Geometry check sheet. Reference: the model listing, model coordinates, mm. Face numbers are marked on the shaded views. A direction names the side the tool comes from. Give positions to 0.01 mm unless a question says otherwise; leave off trailing zeros. Write each loop counter-clockwise with the first axis right and the second up, starting at its lowest first coordinate (ties: lowest second). Pieces come first, ordered by that corner, then holes. Notation, with made-up numbers: M 85.5,-35 L 136.5,-35 A26 cw 136.5,-17 Z; hole C 51,10 d2. An arc over 180 degrees is marked long. One line per item, written item: value. Start each with the question number.
1. Scan lines: line 1 (X direction, y = 54, z = -15); line 2 (Y direction, x = 11, z = -24.5); line 3 (Z direction, x = 13.25, y = 60). Record each from-to range of solid material in increasing order.
2. Gauge pin test, flat ends, axial feed: pin 1 (1 mm diameter, centred on y = 41.5, z = -19, fed in from +X); pin 2 (10 mm diameter, centred on x = 13.5, y = 56.5, fed in from +Z); pin 3 (1.5 mm diameter, centred on x = 20, y = 50, fed in from +Z). Record the tip position at first contact, or that the pin passes through.
3. Tool access check on the marked faces 4 and 5. Record the directions out of +Z, -Z, +X, -X, +Y, -Y that give a thin tool (end or side, any length) a straight path to the whole face; none if there is none.
4. Cross-section at A-A on x = 15. Record the cut outline in (y, z), then the cut area to 3 significant figures.
5. Cross-section at C-C on x = 26. Record the cut outline in (y, z), then the cut area to 3 significant figures.
6. Cross-section at B-B on z = -26. Record the cut outline in (x, y), then the cut area to 3 significant figures.
7. Cross-section at D-D on z = -10.25. Record the cut outline in (x, y).
8. Release check for a two-part mould opening along X. For the marked faces 1, 2 and 3 record: pulls with the +X half, pulls with the -X half, needs draft (parallel to the pull), parting line crosses it, or undercut.
from build123d import *

# Parameters (mm, degrees)
IZIM1_W                     = 30
IZIM1_H                     = 30
Y_KSEKLIK_EKSTR_ZYON1_DEPTH = 40
IZIM2_R                     = 1.5
KES_EKSTR_ZYON1_DEPTH       = 40
IZIM3_R                     = 10
IZIM3_R_2                   = 5.25
Y_KSEKLIK_EKSTR_ZYON2_DEPTH = 40
IZIM4_W                     = 30
IZIM4_H                     = 30
KES_EKSTR_ZYON2_DEPTH       = 32
KES_EKSTR_ZYON3_START       = -10
IZIM5_R                     = 10
KES_EKSTR_ZYON3_DEPTH       = 10
KES_EKSTR_ZYON4_START       = -30
IZIM6_R                     = 5.25
KES_EKSTR_ZYON4_DEPTH       = 30


with BuildPart() as part:
    # Çizim1 → Yükseklik-Ekstrüzyon1 (new body)
    with BuildSketch(Plane(origin=(0, 0, 0), x_dir=(1, 0, 0), z_dir=(0, 1, 0))):
        with Locations((15, 15)):
            Rectangle(IZIM1_W, IZIM1_H)
    extrude(amount=Y_KSEKLIK_EKSTR_ZYON1_DEPTH)

    # Çizim2 → Kes-Ekstrüzyon1 (cut)
    with BuildSketch(Plane(origin=(0, 40, 0), x_dir=(1, 0, 0), z_dir=(0, 1, 0))):
        with Locations(Location((4, 26, 0), (0, 0, 270))):
            Circle(IZIM2_R)
        with Locations(Location((26, 26, 0), (0, 0, 270))):
            Circle(IZIM2_R)
        with Locations(Location((26, 4, 0), (0, 0, 270))):
            Circle(IZIM2_R)
        with Locations(Location((4, 4, 0), (0, 0, 270))):
            Circle(IZIM2_R)
    extrude(amount=-KES_EKSTR_ZYON1_DEPTH, mode=Mode.SUBTRACT)

    # Çizim3 → Yükseklik-Ekstrüzyon2 (add)
    with BuildSketch(Plane(origin=(0, 40, 0), x_dir=(1, 0, 0), z_dir=(0, 1, 0))):
        with Locations(Location((15, 15, 0), (0, 0, 90))):
            Circle(IZIM3_R)
        with Locations(Location((15, 15, 0), (0, 0, 270))):
            Circle(IZIM3_R_2, mode=Mode.SUBTRACT)
    extrude(amount=Y_KSEKLIK_EKSTR_ZYON2_DEPTH)

    # Çizim4 → Kes-Ekstrüzyon2 (cut)
    with BuildSketch(Plane.XZ):
        with Locations((15, -15)):
            Rectangle(IZIM4_W, IZIM4_H)
    extrude(amount=-KES_EKSTR_ZYON2_DEPTH, mode=Mode.SUBTRACT)

    # Çizim5 → Kes-Ekstrüzyon3 (cut)
    with BuildSketch(Plane(origin=(0, 80, 0), x_dir=(1, 0, 0), z_dir=(0, 1, 0)).offset(KES_EKSTR_ZYON3_START)):
        with Locations(Location((15, 15, 0), (0, 0, 90))):
            Circle(IZIM5_R)
    extrude(amount=KES_EKSTR_ZYON3_DEPTH, mode=Mode.SUBTRACT)

    # Çizim6 → Kes-Ekstrüzyon4 (cut)
    with BuildSketch(Plane(origin=(0, 40, 0), x_dir=(1, 0, 0), z_dir=(0, 1, 0)).offset(KES_EKSTR_ZYON4_START)):
        with Locations(Location((15, 15, 0), (0, 0, 270))):
            Circle(IZIM6_R)
    extrude(amount=KES_EKSTR_ZYON4_DEPTH, mode=Mode.SUBTRACT)


solid = part.part
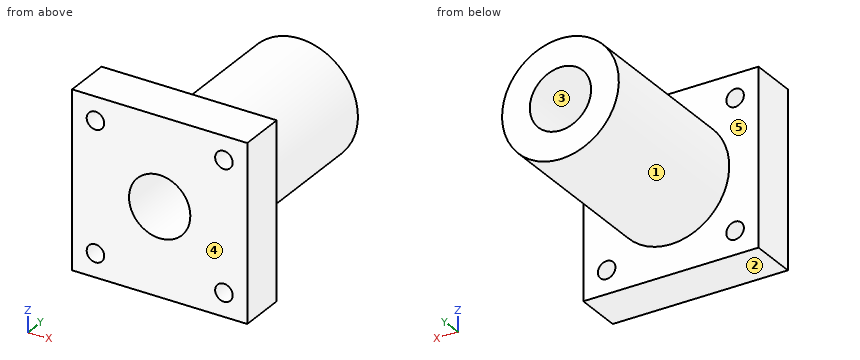
Report:
1. line 1: x = 5 to 9.75, 20.25 to 25
1. line 2: y = 32 to 40
1. line 3: z = -24.85 to -19.95, -10.05 to -5.15
2. pin 1: stops at x = 24.37
2. pin 2: stops at z = -5
2. pin 3: stops at z = -5.95
3. face 4: +Z, -Z, +X, -X, -Y
3. face 5: +Y
4. outline: M 32,-30 L 40,-30 L 40,-25 L 70,-25 L 70,-20.25 L 32,-20.25 Z; M 32,-9.75 L 70,-9.75 L 70,-5 L 40,-5 L 40,0 L 32,0 Z
4. area: 441 mm^2
5. outline: M 32,-30 L 40,-30 L 40,-27.5 L 32,-27.5 Z; M 32,-24.5 L 40,-24.5 L 40,-5.5 L 32,-5.5 Z; M 32,-2.5 L 40,-2.5 L 40,0 L 32,0 Z
5. area: 192 mm^2
6. outline: M 0,32 L 2.5,32 L 2.5,40 L 0,40 Z; M 5.5,32 L 24.5,32 L 24.5,40 L 5.5,40 Z; M 27.5,32 L 30,32 L 30,40 L 27.5,40 Z
6. area: 192 mm^2
7. outline: M 0,32 L 12.76,32 L 12.76,70 L 6.2,70 L 6.2,40 L 0,40 Z; M 17.24,32 L 30,32 L 30,40 L 23.8,40 L 23.8,70 L 17.24,70 Z
8. face 1: parting line crosses it
8. face 2: needs draft
8. face 3: undercut
